Work out the finished part from the listing and answer in its coordinate system (mm). A direction names the side the tool comes from. Coordinates: 2 decimals unless noted, no trailing zeros. Write each loop counter-clockwise with the first axis right and the second up, starting at its lowest first coordinate (ties: lowest second). Pieces come first, ordered by that corner, then holes. Notation, with made-up numbers: (12, 66.5) - (67, 66.5) arc R9 ccw to (67, 83.5) - close; hole circle Ø5 at (-31.5, -34.5). An arc over 180 degrees is marked (long way). Use one line per item in the form item = value. Start each with the question number.
Item 1: For faces 1 (the cylindrical face through (0.14, 49.32, -22.23)), 2 (the cylindrical face through (-16.8, 1.25, -53.36)), 3 (the cylindrical face through (77.784, 18.783, 20.271)), determine the directions among +Z, -Z, +X, -X, +Y, -Y from which every point of the face is accessible in a straight line to the end or side of a thin tool.
Item 2: Determine the mould class of faces 4 (the conical face through (37.47, 42.04, -9.6)), 5 (the cylindrical face through (-19.54, 18.78, -69.39)), 6 (the conical face through (31.56, 32.97, -40.23)) for opening direction Y: released by +Y, released by -Y, zero draft, split by the parting line, or undercut.
Item 3: A cutting plane is placed at B-B (z = 0). Give the number of separate pieces and of enclosed holes in the cut face, then the cut area to 3 significant figures.
Item 4: Given pin 1 (9.5 mm diameter, centred on x = -73.6, z = -19.72, fed in from +Y); pin 2 (2 mm diameter, centred on x = 65.5, y = 30, fed in from +Z); pin 3 (10 mm diameter, centred on y = 34.5, z = -65.5, fed in from +X); pin 4 (4 mm diameter, centred on y = 42, z = -66.5, fed in from +X), each flat-ended and moving along its own axis, determine where each tip first touches the part or whether it passes through.
Item 5: Consider probe 1 along X at (y, z) = (48, 15.5); probe 2 along X at (y, z) = (30.5, -21.5); probe 3 along X at (y, z) = (9.5, -72). Determine where each line is inside the solid, lowest interval first.
Item 6: A cutting plane is placed at A-A (x = -74.5). Write down the section's boundary in (y, z), then the cut area to 3 significant figures.
from build123d import *

# Parameters (mm, degrees)
F_5_16_CLEARANCE_HOLE1_D         = 8.4328
CIRPATTERN1_COUNT                = 12
F_1_2_0_5_DIAMETER_HOLE1_D       = 12.7
F_1_1_5_DIAMETER_HOLE1_D         = 38.1
F_1_1_5_DIAMETER_HOLE1_DEPTH     = 19.05
CIRPATTERN2_COUNT                = 6
CIRPATTERN3_COUNT                = 2
F_1_8_0_125_DIAMETER_HOLE1_D     = 3.175
F_1_8_0_125_DIAMETER_HOLE1_DEPTH = 6.35
F_1_8_0_125_DIAMETER_HOLE1_TIP   = 0.953866233


with BuildPart() as part:
    # Sketch1 → Revolve1 (revolve)
    with BuildSketch(Plane.XY, mode=Mode.PRIVATE) as revolve1_sk:
        Polygon((-55.9435, 0), (-88.9, 0), (-88.9, 38.1), (-50.8, 38.1), (-31.75, 57.15), (0, 57.15), (0, 31.75), (-31.75, 31.75), (-31.75, 19.05), (-50.8, 19.05), (-50.8, 0), (-52.3875, 0), (-52.3875, 2.54), (-55.9435, 2.54), align=None)
    revolve(revolve1_sk.sketch.rotate(Axis((0, 0, 0), (0, 1, 0)), 270), axis=Axis((0, 0, 0), (0, 1, 0)))

    # 5/16 Clearance Hole1 (through all)
    with Locations(Plane(origin=(0, 38.1, 0), x_dir=(1, 0, 0), z_dir=(0, 1, 0))):
        with Locations((-73.603547963, -19.722011237)):
            f_5_16_clearance_hole1 = Hole(F_5_16_CLEARANCE_HOLE1_D / 2)

    # CirPattern1: 5/16 Clearance Hole1 ×12 about axis
    cirpattern1_axis = Axis((0, 0, 0), (0, 1, 0))
    for i in range(1, CIRPATTERN1_COUNT):
        add(f_5_16_clearance_hole1.rotate(cirpattern1_axis, i * 360 / CIRPATTERN1_COUNT), mode=Mode.SUBTRACT)

    # 1/2 (0.5) Diameter Hole1 (through all)
    with Locations(Plane(origin=(0, 57.15, 0), x_dir=(1, 0, 0), z_dir=(0, 1, 0))):
        with Locations((0, 0)):
            Hole(F_1_2_0_5_DIAMETER_HOLE1_D / 2)

    # Sketch11 → 1/2 NPT Tapped Hole1 (revolve, cut)
    with BuildSketch(Plane(origin=(41.275, 47.625, 0), x_dir=(-0.707106781186546, 0.707106781186549, 0), z_dir=(0, 0, 1))):
        Polygon((0, 0), (0, 125.723585695), (8.9281, 125.723585695), (8.9281, 13.462), (9.479726792, 13.462), (9.8827971, 0), align=None)
    revolve(axis=Axis((45.765128061, 52.115128061, 0), (-0.707106781186549, -0.707106781186546, 0)), mode=Mode.SUBTRACT)

    # 1 (1.5) Diameter Hole1
    with Locations(Plane(origin=(0, 57.15, 0), x_dir=(1, 0, 0), z_dir=(0, 1, 0))):
        with Locations((-23.8125, -41.244459855)):
            f_1_1_5_diameter_hole1 = Hole(F_1_1_5_DIAMETER_HOLE1_D / 2, depth=F_1_1_5_DIAMETER_HOLE1_DEPTH)

    # Sketch19 → 3/8 NPT Tapped Hole1 (revolve, cut)
    with BuildSketch(Plane(origin=(-23.8125, 38.1, 41.244459855), x_dir=(0, 0, 1), z_dir=(1, 0, 0))):
        Polygon((0, 0), (0, 26.640582582), (7.1374, 22.352), (7.1374, 10.414), (7.653732494, 10.414), (7.9655416, 0), align=None)
    f_3_8_npt_tapped_hole1 = revolve(axis=Axis((-23.8125, 44.45, 41.244459855), (0, -1, 0)), mode=Mode.SUBTRACT)

    # Sketch21 → 1/4 (0.25) Diameter Hole1 (revolve, cut)
    with BuildSketch(Plane(origin=(21.997045256, 57.15, -12.7), x_dir=(0, 0, 1), z_dir=(1, 0, 0))):
        Polygon((0, 0), (0, 17.782732465), (3.175, 15.875), (3.175, 0), align=None)
    f_1_4_0_25_diameter_hole1 = revolve(axis=Axis((21.997045256, 63.5, -12.7), (0, -1, 0)), mode=Mode.SUBTRACT)

    # CirPattern2: 1/4 (0.25) Diameter Hole1 ×6 about axis
    cirpattern2_axis = Axis((0, 0, 0), (0, 1, 0))
    for i in range(1, CIRPATTERN2_COUNT):
        add(f_1_4_0_25_diameter_hole1.rotate(cirpattern2_axis, i * 360 / CIRPATTERN2_COUNT), mode=Mode.SUBTRACT)

    # CirPattern3: 1 (1.5) Diameter Hole1, 3/8 NPT Tapped Hole1 ×2 about axis
    cirpattern3_axis = Axis((0, 0, 0), (0, 1, 0))
    add([f_1_1_5_diameter_hole1.rotate(cirpattern3_axis, i * 360 / CIRPATTERN3_COUNT) for i in range(1, CIRPATTERN3_COUNT)], mode=Mode.SUBTRACT)
    add([f_3_8_npt_tapped_hole1.rotate(cirpattern3_axis, i * 360 / CIRPATTERN3_COUNT) for i in range(1, CIRPATTERN3_COUNT)], mode=Mode.SUBTRACT)

    # 1/8 (0.125) Diameter Hole1
    with Locations(Plane(origin=(0, 19.05, 0), x_dir=(-1, 0, 0), z_dir=(0, -1, 0))):
        with Locations((0, 44.45)):
            Hole(F_1_8_0_125_DIAMETER_HOLE1_D / 2, depth=F_1_8_0_125_DIAMETER_HOLE1_DEPTH)
            with Locations((0, 0, -(F_1_8_0_125_DIAMETER_HOLE1_DEPTH + F_1_8_0_125_DIAMETER_HOLE1_TIP / 2))):  # 118° drill point
                Cone(0, F_1_8_0_125_DIAMETER_HOLE1_D / 2, F_1_8_0_125_DIAMETER_HOLE1_TIP, mode=Mode.SUBTRACT)


solid = part.part
Answer:
q1.face_1 = +Y
q1.face_2 = -Y
q1.face_3 = +Y, -Y
q2.face_4 = undercut
q2.face_5 = zero draft
q2.face_6 = released by +Y
q3.separate_pieces = 3
q3.enclosed_holes = 0
q3.area = 4,820 mm²
q4.pin_1 = 38.1
q4.pin_2 = 61.18
q4.pin_3 = 65.14
q4.pin_4 = through
q5.probe_1 = -37.85 to -23.49, -20.5 to 20.5, 23.49 to 37.85
q5.probe_2 = -86.26 to -77.43, -69.78 to -23.36, 23.36 to 69.78, 77.43 to 86.26
q5.probe_3 = -52.15 to -23.62, -15.82 to 15.82, 23.62 to 52.15
q6.outline = (0, -48.51) - (38.1, -48.51) - (38.1, -23.84) - (0, -23.84) - close; (0, -15.6) - (38.1, -15.6) - (38.1, 15.6) - (0, 15.6) - close; (0, 23.84) - (38.1, 23.84) - (38.1, 48.51) - (0, 48.51) - close
q6.area = 3,070 mm²
